CAD build for the part. Positions are in the model's coordinates, mm. A direction names the side the tool comes from. Coordinates: 2 decimals unless noted, no trailing zeros. Loops run counter-clockwise (first coordinate to the right, second up) from the corner with the lowest first, then second, coordinate; pieces in that order, holes last. Notation, with made-up numbers: (40.25, 13.5) -> (62.25, 13.5) arc R30 cw to (62.25, 38.5) -> close; hole circle Ø8 at (10, 30.25). An arc over 180 degrees is marked (long way). Answer as CSV lines item,"result". Start each with the question number.
from build123d import *

# Parameters (mm, degrees)
SKETCH1_W            = 106.5
SKETCH1_H            = 74.5
BOSS_EXTRUDE1_DEPTH  = 3
SKETCH2_W            = 6.93
SKETCH2_H            = 1.85
BOSS_EXTRUDE2_DEPTH  = 3
SKETCH3_W            = 6.93
SKETCH3_H            = 1.85
CUT_EXTRUDE1_DEPTH   = 1.07
SKETCH4_W            = 5
SKETCH4_H            = 64.5
SKETCH4_W_2          = 78.5
SKETCH4_H_2          = 15
CUT_EXTRUDE2_DEPTH   = 3
SKETCH5_R            = 3.5
CUT_EXTRUDE3_DEPTH   = 3
BOSS_EXTRUDE5_DEPTH  = 5
SKETCH9_R            = 3
SKETCH9_R_2          = 1.5
BOSS_EXTRUDE6_DEPTH  = 2
SKETCH10_W           = 15
SKETCH10_H           = 21
BOSS_EXTRUDE7_DEPTH  = 1
BOSS_EXTRUDE8_DEPTH  = 2
SKETCH12_W           = 5
SKETCH12_H           = 5
CUT_EXTRUDE4_DEPTH   = 4
SKETCH14_W           = 4
SKETCH14_H           = 75.31405771
CUT_EXTRUDE5_DEPTH   = 10
SKETCH15_R           = 3
SKETCH15_R_2         = 1.5
BOSS_EXTRUDE9_DEPTH  = 3
SKETCH16_R           = 1.5
CUT_EXTRUDE6_DEPTH   = 3
SKETCH17_R           = 1.5
CUT_EXTRUDE7_DEPTH   = 3
SKETCH18_W           = 7
SKETCH18_H           = 2
CUT_EXTRUDE8_DEPTH   = 3
SKETCH19_R           = 1.5
CUT_EXTRUDE9_DEPTH   = 3
SKETCH20_W           = 3
SKETCH20_H           = 74.5
CUT_EXTRUDE10_DEPTH  = 8
SKETCH21_W           = 1
SKETCH21_H           = 15
BOSS_EXTRUDE10_DEPTH = 3


with BuildPart() as part:
    # Sketch1 → Boss-Extrude1 (new body)
    with BuildSketch(Plane(origin=(0, 0, 0), x_dir=(1, 0, 0), z_dir=(0, 1, 0))):
        Rectangle(SKETCH1_W, SKETCH1_H)
    extrude(amount=BOSS_EXTRUDE1_DEPTH)

    # Sketch2 → Boss-Extrude2 (add)
    with BuildSketch(Plane(origin=(0, 3, 0), x_dir=(1, 0, 0), z_dir=(0, 1, 0))):
        with Locations((-43.8, 38.175)):
            Rectangle(SKETCH2_W, SKETCH2_H)
        with Locations((38.315, 38.175)):
            Rectangle(SKETCH2_W, SKETCH2_H)
    extrude(amount=-BOSS_EXTRUDE2_DEPTH)

    # Sketch3 → Cut-Extrude1 (cut)
    with BuildSketch(Plane(origin=(0, 3, 0), x_dir=(1, 0, 0), z_dir=(0, 1, 0))):
        with Locations((-43.8, 38.175)):
            Rectangle(SKETCH3_W, SKETCH3_H)
        with Locations((38.315, 38.175)):
            Rectangle(SKETCH3_W, SKETCH3_H)
    extrude(amount=-CUT_EXTRUDE1_DEPTH, mode=Mode.SUBTRACT)

    # Sketch4 → Cut-Extrude2 (cut)
    with BuildSketch(Plane(origin=(0, 3, 0), x_dir=(1, 0, 0), z_dir=(0, 1, 0))):
        with Locations((-50.75, 0)):
            Rectangle(SKETCH4_W, SKETCH4_H)
        with Locations((0, -29.75)):
            Rectangle(SKETCH4_W_2, SKETCH4_H_2)
    extrude(amount=-CUT_EXTRUDE2_DEPTH, mode=Mode.SUBTRACT)

    # Sketch5 → Cut-Extrude3 (cut)
    with BuildSketch(Plane(origin=(0, 3, 0), x_dir=(1, 0, 0), z_dir=(0, 1, 0))):
        with Locations((-53.25, -37.25)):
            Circle(SKETCH5_R)
        with Locations((53.25, -37.25)):
            Circle(SKETCH5_R)
        with Locations((53.25, 37.25)):
            Circle(SKETCH5_R)
        with Locations((-53.25, 37.25)):
            Circle(SKETCH5_R)
    extrude(amount=-CUT_EXTRUDE3_DEPTH, mode=Mode.SUBTRACT)

    # Sketch6 → Boss-Extrude5 (add)
    with BuildSketch(Plane(origin=(0, 3, 0), x_dir=(1, 0, 0), z_dir=(0, 1, 0))):
        with BuildLine():
            Line((-29.091687605, 12.75), (-32.408312395, 12.75))
            ThreePointArc((-32.408312395, 12.75), (-32.871320344, 12.371320344), (-33.25, 11.908312395))
            Line((-33.25, 11.908312395), (-33.25, 8.591687605))
            ThreePointArc((-33.25, 8.591687605), (-30.382155065, 7.272637055), (-27.921572875, 9.25))
            Line((-27.921572875, 9.25), (-29.631966011, 9.25))
            ThreePointArc((-29.631966011, 9.25), (-32.25, 10.25), (-29.631966011, 11.25))
            Line((-29.631966011, 11.25), (-27.921572875, 11.25))
            ThreePointArc((-27.921572875, 11.25), (-28.384580824, 12.09520788), (-29.091687605, 12.75))
        make_face()
        with BuildLine():
            Line((-33.25, 8.591687605), (-33.25, 11.908312395))
            ThreePointArc((-33.25, 11.908312395), (-33.75, 10.25), (-33.25, 8.591687605))
        make_face()
        with BuildLine():
            ThreePointArc((-29.091687605, 12.75), (-30.75, 13.25), (-32.408312395, 12.75))
            Line((-32.408312395, 12.75), (-29.091687605, 12.75))
        make_face()
        with BuildLine():
            ThreePointArc((-27.921572875, -12.75), (-30.382155065, -10.772637055), (-33.25, -12.091687605))
            Line((-33.25, -12.091687605), (-33.25, -15.408312395))
            ThreePointArc((-33.25, -15.408312395), (-32.871320344, -15.871320344), (-32.408312395, -16.25))
            Line((-32.408312395, -16.25), (-29.091687605, -16.25))
            ThreePointArc((-29.091687605, -16.25), (-28.384580824, -15.59520788), (-27.921572875, -14.75))
            Line((-27.921572875, -14.75), (-29.631966011, -14.75))
            ThreePointArc((-29.631966011, -14.75), (-32.25, -13.75), (-29.631966011, -12.75))
            Line((-29.631966011, -12.75), (-27.921572875, -12.75))
        make_face()
        with BuildLine():
            Line((-33.25, -15.408312395), (-33.25, -12.091687605))
            ThreePointArc((-33.25, -12.091687605), (-33.75, -13.75), (-33.25, -15.408312395))
        make_face()
        with BuildLine():
            Line((-29.091687605, -16.25), (-32.408312395, -16.25))
            ThreePointArc((-32.408312395, -16.25), (-30.75, -16.75), (-29.091687605, -16.25))
        make_face()
        with BuildLine():
            Line((22.75, -15.408312395), (22.75, -12.091687605))
            ThreePointArc((22.75, -12.091687605), (19.882155065, -10.772637055), (17.421572875, -12.75))
            Line((17.421572875, -12.75), (19.131966011, -12.75))
            ThreePointArc((19.131966011, -12.75), (20.785233135, -12.348741462), (21.75, -13.75))
            ThreePointArc((21.75, -13.75), (20.785233135, -15.151258538), (19.131966011, -14.75))
            Line((19.131966011, -14.75), (17.421572875, -14.75))
            ThreePointArc((17.421572875, -14.75), (17.884580824, -15.59520788), (18.591687605, -16.25))
            Line((18.591687605, -16.25), (21.908312395, -16.25))
            ThreePointArc((21.908312395, -16.25), (22.371320344, -15.871320344), (22.75, -15.408312395))
        make_face()
        with BuildLine():
            Line((21.908312395, -16.25), (18.591687605, -16.25))
            ThreePointArc((18.591687605, -16.25), (20.25, -16.75), (21.908312395, -16.25))
        make_face()
        with BuildLine():
            ThreePointArc((23.25, -13.75), (23.122281323, -12.883974596), (22.75, -12.091687605))
            Line((22.75, -12.091687605), (22.75, -15.408312395))
            ThreePointArc((22.75, -15.408312395), (23.122281323, -14.616025404), (23.25, -13.75))
        make_face()
        with BuildLine():
            Line((21.908312395, 12.75), (18.591687605, 12.75))
            ThreePointArc((18.591687605, 12.75), (17.884580824, 12.09520788), (17.421572875, 11.25))
            Line((17.421572875, 11.25), (19.131966011, 11.25))
            ThreePointArc((19.131966011, 11.25), (20.785233135, 11.651258538), (21.75, 10.25))
            ThreePointArc((21.75, 10.25), (20.785233135, 8.848741462), (19.131966011, 9.25))
            Line((19.131966011, 9.25), (17.421572875, 9.25))
            ThreePointArc((17.421572875, 9.25), (19.882155065, 7.272637055), (22.75, 8.591687605))
            Line((22.75, 8.591687605), (22.75, 11.908312395))
            ThreePointArc((22.75, 11.908312395), (22.371320344, 12.371320344), (21.908312395, 12.75))
        make_face()
        with BuildLine():
            ThreePointArc((23.25, 10.25), (23.122281323, 11.116025404), (22.75, 11.908312395))
            Line((22.75, 11.908312395), (22.75, 8.591687605))
            ThreePointArc((22.75, 8.591687605), (23.122281323, 9.383974596), (23.25, 10.25))
        make_face()
        with BuildLine():
            ThreePointArc((21.908312395, 12.75), (20.25, 13.25), (18.591687605, 12.75))
            Line((18.591687605, 12.75), (21.908312395, 12.75))
        make_face()
    extrude(amount=BOSS_EXTRUDE5_DEPTH)

    # Sketch9 → Boss-Extrude6 (add)
    with BuildSketch(Plane(origin=(0, 3, 0), x_dir=(1, 0, 0), z_dir=(0, 1, 0))):
        with Locations((38.25, -7.75)):
            Circle(SKETCH9_R)
        with Locations((38.25, -7.75)):
            Circle(SKETCH9_R_2, mode=Mode.SUBTRACT)
    extrude(amount=BOSS_EXTRUDE6_DEPTH)

    # Sketch10 → Boss-Extrude7 (add)
    with BuildSketch(Plane(origin=(0, 3, 0), x_dir=(1, 0, 0), z_dir=(0, 1, 0))):
        with Locations((-2.5, 21.75)):
            Rectangle(SKETCH10_W, SKETCH10_H)
        Polygon((-15, 6.25), (-15, 37.25), (-17, 37.25), (-17, 4.25), (12, 4.25), (12, 37.25), (10, 37.25), (10, 6.25), align=None)
    extrude(amount=BOSS_EXTRUDE7_DEPTH)

    # Sketch11 → Boss-Extrude8 (add)
    with BuildSketch(Plane(origin=(0, 4, 0), x_dir=(1, 0, 0), z_dir=(0, 1, 0))):
        Polygon((-15, 37.25), (-17, 37.25), (-17, 4.25), (12, 4.25), (12, 37.25), (10, 37.25), (10, 6.25), (-15, 6.25), align=None)
    extrude(amount=BOSS_EXTRUDE8_DEPTH)

    # Sketch12 → Cut-Extrude4 (cut)
    with BuildSketch(Plane(origin=(0, 3, 0), x_dir=(1, 0, 0), z_dir=(0, 1, 0))):
        with Locations((-50.75, 34.75)):
            Rectangle(SKETCH12_W, SKETCH12_H)
        with Locations((-50.75, -34.75)):
            Rectangle(SKETCH12_W, SKETCH12_H)
    extrude(amount=-CUT_EXTRUDE4_DEPTH, mode=Mode.SUBTRACT)

    # Sketch14 → Cut-Extrude5 (cut)
    with BuildSketch(Plane(origin=(0, 3, 0), x_dir=(1, 0, 0), z_dir=(0, 1, 0))):
        with Locations((51.75, 0.407028855)):
            Rectangle(SKETCH14_W, SKETCH14_H)
    extrude(amount=-CUT_EXTRUDE5_DEPTH, mode=Mode.SUBTRACT)

    # Sketch15 → Boss-Extrude9 (add)
    with BuildSketch(Plane(origin=(0, 3, 0), x_dir=(1, 0, 0), z_dir=(0, 1, 0))):
        with Locations((15.5, 20.75)):
            Circle(SKETCH15_R)
        with Locations((15.5, 20.75)):
            Circle(SKETCH15_R_2, mode=Mode.SUBTRACT)
        with Locations((-20.5, 20.75)):
            Circle(SKETCH15_R)
        with Locations((-20.5, 20.75)):
            Circle(SKETCH15_R_2, mode=Mode.SUBTRACT)
    extrude(amount=BOSS_EXTRUDE9_DEPTH)

    # Sketch16 → Cut-Extrude6 (cut)
    with BuildSketch(Plane(origin=(0, 3, 0), x_dir=(1, 0, 0), z_dir=(0, 1, 0))):
        with Locations((15.5, 20.75)):
            Circle(SKETCH16_R)
        with Locations((-20.5, 20.75)):
            Circle(SKETCH16_R)
    extrude(amount=-CUT_EXTRUDE6_DEPTH, mode=Mode.SUBTRACT)

    # Sketch17 → Cut-Extrude7 (cut)
    with BuildSketch(Plane(origin=(0, 3, 0), x_dir=(1, 0, 0), z_dir=(0, 1, 0))):
        with Locations((38.25, -7.75)):
            Circle(SKETCH17_R)
    extrude(amount=-CUT_EXTRUDE7_DEPTH, mode=Mode.SUBTRACT)

    # Sketch18 → Cut-Extrude8 (cut)
    with BuildSketch(Plane(origin=(0, 6, 0), x_dir=(1, 0, 0), z_dir=(0, 1, 0))):
        with Locations((6.5, 5.25)):
            Rectangle(SKETCH18_W, SKETCH18_H)
        with Locations((-11.5, 5.25)):
            Rectangle(SKETCH18_W, SKETCH18_H)
    extrude(amount=-CUT_EXTRUDE8_DEPTH, mode=Mode.SUBTRACT)

    # Sketch19 → Cut-Extrude9 (cut)
    with BuildSketch(Plane(origin=(0, 3, 0), x_dir=(1, 0, 0), z_dir=(0, 1, 0))):
        with Locations((41.035, -34.25)):
            Circle(SKETCH19_R)
        with Locations((-44.73, -34.25)):
            Circle(SKETCH19_R)
    extrude(amount=-CUT_EXTRUDE9_DEPTH, mode=Mode.SUBTRACT)

    # Sketch20 → Cut-Extrude10 (cut)
    with BuildSketch(Plane(origin=(0, 3, 0), x_dir=(1, 0, 0), z_dir=(0, 1, 0))):
        with Locations((48.25, 0)):
            Rectangle(SKETCH20_W, SKETCH20_H)
    extrude(amount=-CUT_EXTRUDE10_DEPTH, mode=Mode.SUBTRACT)

    # Sketch21 → Boss-Extrude10 (add)
    with BuildSketch(Plane(origin=(0, 3, 0), x_dir=(1, 0, 0), z_dir=(0, 1, 0))):
        with Locations((38.75, -29.75)):
            Rectangle(SKETCH21_W, SKETCH21_H)
    extrude(amount=-BOSS_EXTRUDE10_DEPTH)


solid = part.part
Item 1: Saw through at B-B (z = 27). Write the cut outline in (x, y), plus the area to 3 significant figures.
Item 2: Flat gauge pins, fed straight in: pin 1 Ø1 at (x, y) = (23.5, 6) entering from +Z; pin 2 Ø4 at (x, y) = (32, 4.5) entering from -Z; pin 3 Ø10 at (x, z) = (20, -17) entering from -Y; pin 4 Ø2.5 at (x, z) = (-30.75, 13.75) entering from +Y. Where does each tip first touch, or does it go through?
Item 3: Two-plate mould, pull along X, no slides. Class faces 1 (the face through (-32.25, 5.46, 13.8)), 2 (the face through (41.78, 1, -38)), 3 (the face through (22, 8, 13)): pulls with the +X half, pulls with the -X half, needs draft (parallel to the pull), parting line crosses it, or undercut.
Item 4: Which spindle directions (+Z, -Z, +X, -X, +Y, -Y) get a long thin tool onto all of the face, cutting with end or side? Do faces 4 (the face through (14, 6, -20)), 5 (the face through (11, 4, -4.25)), 6 (the face through (-17, 4, -21)), 7 (the face through (34.85, 1, -38)), 8 (the face through (-1, 2, 22.25)). Say none if no direction does.
Item 5: Saw through at D-D (z = 7.75). Write the cut outline in (x, y), plus the area to 3 significant figures.
Item 6: Saw through at A-A (x = -20.5). Write the cut outline in (y, z), plus the area to 4 significant figures.
Item 7: Saw through at C-C (z = -20.75). Count the separate pieces of the cut face and the enclosed holes in it, plus the area to 3 significant figures.
Item 8: Wall check: probe 1 along X at (y, z) = (4.65, -10.25); probe 2 along X at (y, z) = (1.9, -20.75); probe 3 along Z at (x, y) = (-20.5, 0.75). Give the ranges that are in metal, low to high.
Geometry check:
1,outline,"(-48.25, 0) -> (-39.25, 0) -> (-39.25, 3) -> (-48.25, 3) -> close; (38.25, 0) -> (46.75, 0) -> (46.75, 3) -> (38.25, 3) -> close"
1,area,"52.5 mm2"
2,pin 1,"z = 14.95"
2,pin 2,"z = -37.25"
2,pin 3,"y = 0"
2,pin 4,"y = 3"
3,face 1,"undercut"
3,face 2,"pulls with the +X half"
3,face 3,"needs draft"
4,face 4,"-Z, +X, -X, +Y"
4,face 5,"+Z, +X, -X, +Y"
4,face 6,"+Z, -Z, +Y"
4,face 7,"-Z, +Y, -Y"
4,face 8,"+Z, +Y, -Y"
5,outline,"(-48.25, 0) -> (36.75, 0) -> (36.75, 5) -> (35.25, 5) -> (35.25, 3) -> (-48.25, 3) -> close; (39.75, 0) -> (46.75, 0) -> (46.75, 3) -> (41.25, 3) -> (41.25, 5) -> (39.75, 5) -> close"
5,area,"282 mm2"
6,outline,"(0, -37.25) -> (3, -37.25) -> (3, -23.75) -> (6, -23.75) -> (6, -22.25) -> (0, -22.25) -> close; (0, -19.25) -> (6, -19.25) -> (6, -17.75) -> (3, -17.75) -> (3, 22.25) -> (0, 22.25) -> close"
6,area,"178.5 mm2"
7,separate pieces,"3"
7,enclosed holes,"0"
7,area,"312 mm2"
8,probe 1,"-33.75 to -32.25, -17 to -15, 10 to 12, 21.75 to 23.25"
8,probe 2,"-48.25 to -22, -19 to 14, 17 to 46.75"
8,probe 3,"-37.25 to -22.25, -19.25 to 22.25"
